Print and shaded views of the part. All mm, measured from the part's lowest x, y and z. Coordinates: 2 decimals unless noted, no trailing zeros. Order: outer loops, then holes, each group sorted by start corner. A loop starts at its lowest first (then second) coordinate and runs counter-clockwise, first axis right, second up. Notation, with made-up numbers: (0.25, -25.75) -> (40.25, -25.75) arc R23 ccw to (40.25, -16.75) -> close; hole circle Ø2 at (39, -19.75). An arc over 180 degrees is marked (long way). Use one line per item in the form item = value. Start each with the question number.
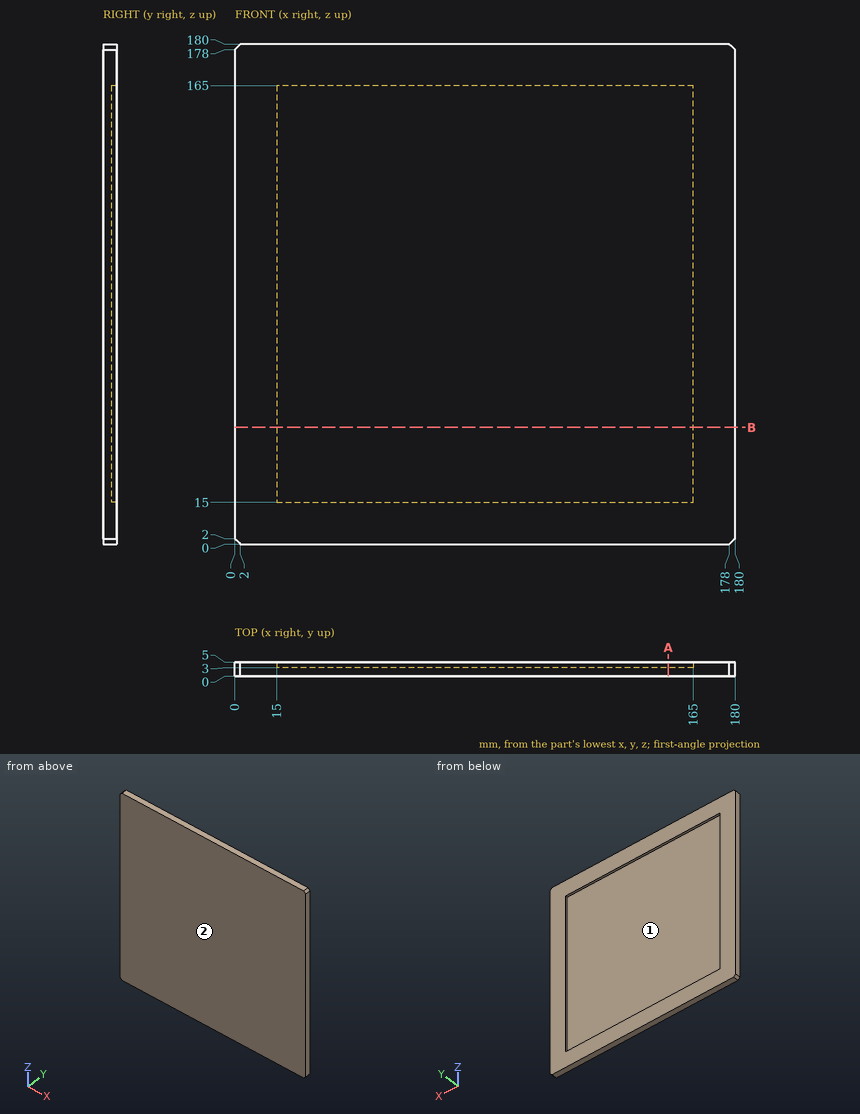
1) Probe L1, parallel to Z at x = 39, y = 3.9; L2, parallel to Y at x = 65.5, z = 37. List the from-to ranges inside material, lowest first.
2) Drop a flat-ended pin along its axis: P1, Ø8, axis at x = 21.5, z = 106.5, coming from the +Y side. Give the stop position or say it passes through.
3) Cut at B-B on z = 42. Give the cut face in (x, y).
4) Cut at A-A on x = 156. Give the cut face in (y, z), then the cut area to 3 significant figures.
5) Two-plate mould, pull along X, no slides. Class the marked faces 1 and 2: released by +X, released by -X, zero draft, split by the parting line, or undercut.
Values follow:
q1.L1 = 0 to 15, 165 to 180
q1.L2 = 0 to 3
q2.P1 = 3
q3.outline = (0, 0) -> (180, 0) -> (180, 5) -> (165, 5) -> (165, 3) -> (15, 3) -> (15, 5) -> (0, 5) -> close
q4.outline = (0, 0) -> (5, 0) -> (5, 15) -> (3, 15) -> (3, 165) -> (5, 165) -> (5, 180) -> (0, 180) -> close
q4.area = 600 mm^2
q5.face_1 = undercut
q5.face_2 = zero draft
